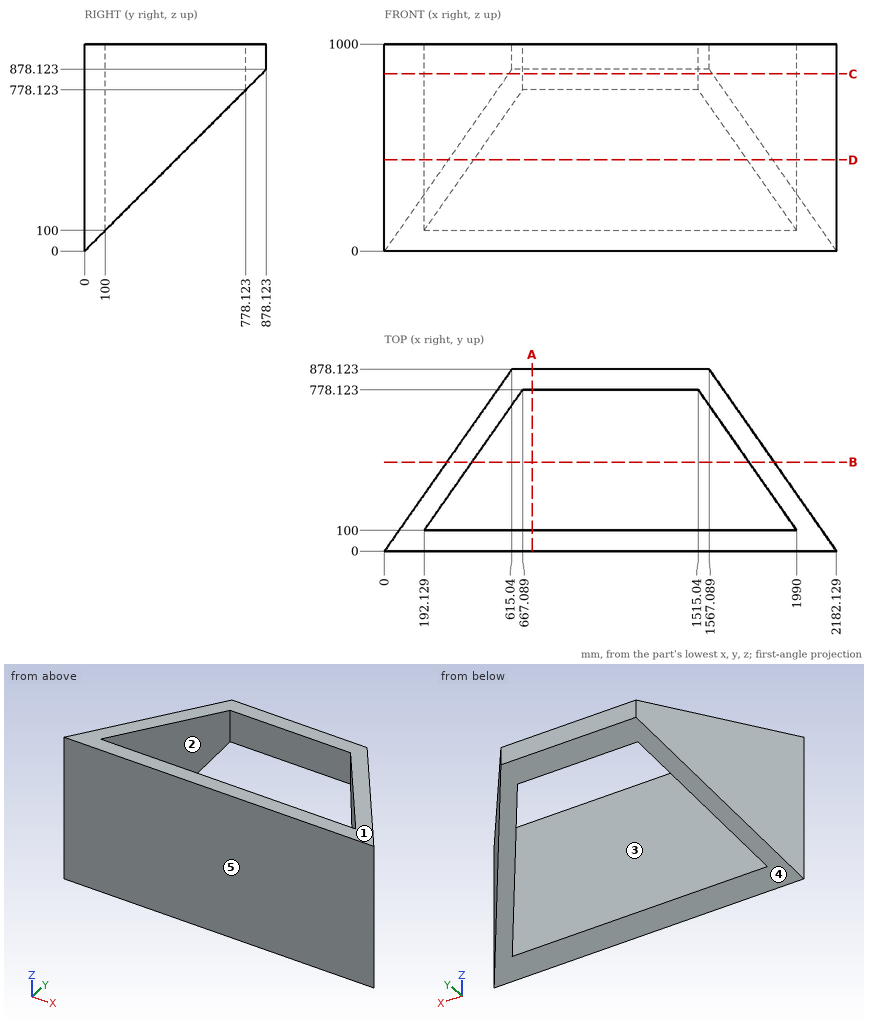
The figure shows three views and two pictorial views of one solid part (mm, origin at its lowest corner). Answer the questions. A direction names the side the tool comes from. Give positions to 0.01 mm unless a question says otherwise; leave off trailing zeros. Loops run counter-clockwise (first coordinate to the right, second up) from the corner with the lowest first, then second, coordinate; pieces in that order, holes last. Notation, with made-up numbers: (18, 11) -> (27, 11) arc R28 ccw to (27, 48) -> close; hole circle Ø4 at (59.5, 43). An arc over 180 degrees is marked (long way). Use a Markdown table: item, result. Add a question column.
1. Section D-D on z = 441 is taken. Determine the outline of the cut face in (x, y).
2. For the marked faces 1 and 2, determine the directions among +Z, -Z, +X, -X, +Y, -Y from which every point of the face is accessible in a straight line to the end or side of a thin tool.
3. Flat-ended cylindrical pins translate along their axes: pin 1 Ø4 at (x, y) = (1555.5, 727.5) entering from -Z; pin 2 Ø4 at (y, z) = (372.5, 768.5) entering from -X; pin 3 Ø1 at (x, z) = (836, 608.5) entering from +Y. Find the tip coordinate at first contact, or state that the pin passes through.
4. Section C-C on z = 856 is taken. Determine the outline of the cut face in (x, y) (1 decimal), and give its area (3 significant figures).
5. Find the intervals of material crossed by probe 1 along Y at (x, z) = (1571.5, 931) (1 decimal); probe 2 along Y at (x, z) = (406, 138); probe 3 along Y at (x, z) = (594, 676.5), in increasing order.
6. Section A-A on x = 713.5 is taken. Determine the outline of the cut face in (y, z), and give its area (3 significant figures).
7. Section B-B on y = 430 is taken. Determine the outline of the cut face in (x, z) (1 decimal).
8. Determine the mould class of the marked faces 3, 4 and 5 for opening direction Y: released by +Y, released by -Y, zero draft, split by the parting line, or undercut.
Results below:
| question | item | result |
|---|---|---|
| 1 | outline | (0, 0) -> (2182.13, 0) -> (1873.25, 441) -> (1751.16, 441) -> (1990, 100) -> (192.13, 100) -> (430.97, 441) -> (308.88, 441) -> close |
| 2 | face 1 | +Z, +X, -X, +Y, -Y |
| 2 | face 2 | +Z, -Z |
| 3 | pin 1 | stops at z = 725.5 |
| 3 | pin 2 | stops at x = 259.5 |
| 3 | pin 3 | stops at y = 100 |
| 4 | outline | (0, 0) -> (2182.1, 0) -> (1582.6, 856) -> (599.5, 856) -> close; hole (192.1, 100) -> (1990, 100) -> (1515, 778.1) -> (667.1, 778.1) -> close |
| 4 | area | 458,000 mm^2 |
| 5 | probe 1 | y = 0 to 100, 697.5 to 871.8 |
| 5 | probe 2 | y = 0 to 100 |
| 5 | probe 3 | y = 0 to 100, 673.77 to 676.5 |
| 6 | outline | (0, 0) -> (100, 100) -> (100, 1000) -> (0, 1000) -> close; (778.12, 778.12) -> (878.12, 878.12) -> (878.12, 1000) -> (778.12, 1000) -> close |
| 6 | area | 112,000 mm^2 |
| 7 | outline | (301.2, 430) -> (423.3, 430) -> (423.3, 1000) -> (301.2, 1000) -> close; (1758.9, 430) -> (1881, 430) -> (1881, 1000) -> (1758.9, 1000) -> close |
| 8 | face 3 | undercut |
| 8 | face 4 | released by +Y |
| 8 | face 5 | released by -Y |
